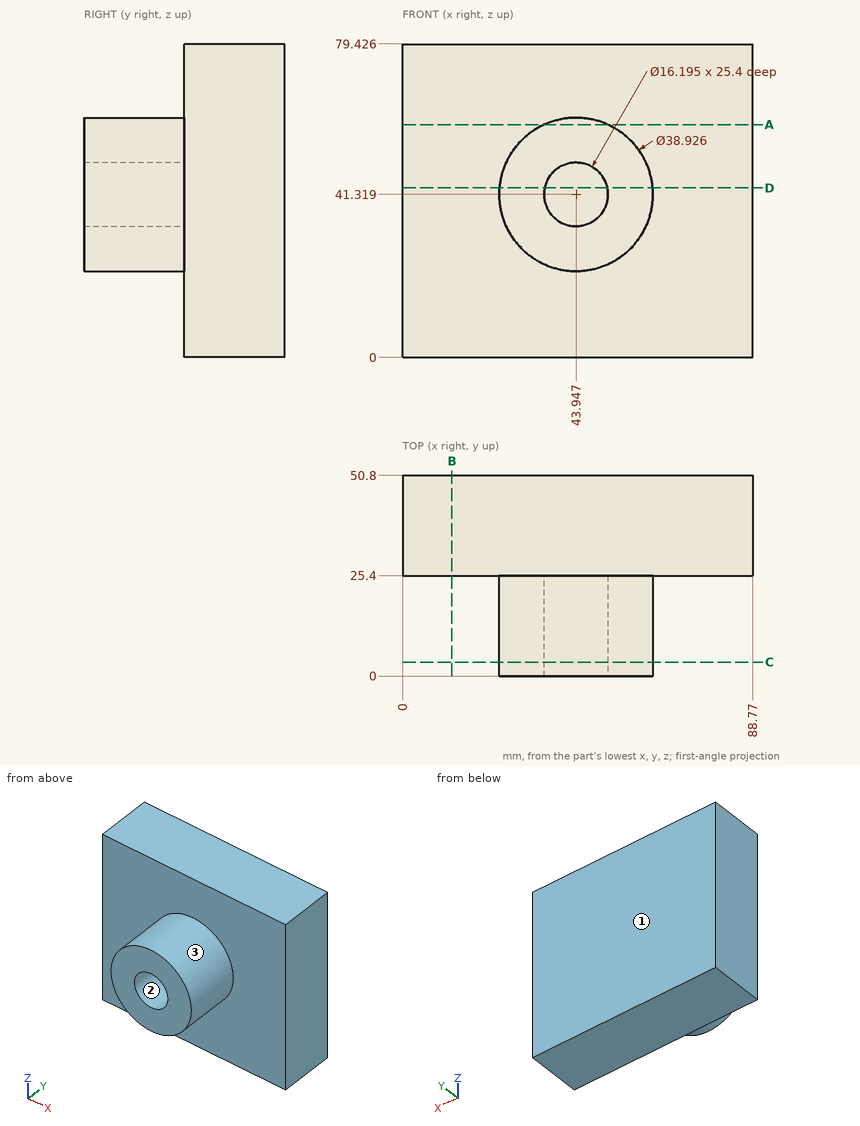
Job drawing, mm, ordinate dimensions from the low corner. One solid piece. Give positions to 0.01 mm unless a question says otherwise; leave off trailing zeros. Loops run counter-clockwise (first coordinate to the right, second up) from the corner with the lowest first, then second, coordinate; pieces in that order, holes last.
Item 1: Pull direction Z, two halves, no side cores. Call the marked faces 1, 2 and 3: released by +Z, released by -Z, zero draft, split by the parting line, or undercut.
Answers follow:
face 1: zero draft
face 2: undercut
face 3: split by the parting line
Item 2: Slice it at D-D, the plane z = 43. List the corners of the cut face in (x, y).
Answers follow:
outline: (0, 25.4) - (24.56, 25.4) - (24.56, 0) - (36.03, 0) - (36.03, 25.4) - (51.87, 25.4) - (51.87, 0) - (63.34, 0) - (63.34, 25.4) - (88.77, 25.4) - (88.77, 50.8) - (0, 50.8) - close
Item 3: Slice it at C-C, the plane y = 3.5. List the corners of the cut face in (x, z) (1 decimal).
Answers follow:
outline: circle Ø38.9 at (43.9, 41.3); hole circle Ø16.2 at (43.9, 41.3)
Item 4: Slice it at B-B, the plane x = 12.5. List the corners of the cut face in (y, z).
Answers follow:
outline: (25.4, 0) - (50.8, 0) - (50.8, 79.43) - (25.4, 79.43) - close
Item 5: Slice it at A-A, the plane z = 59. List the corners of the cut face in (x, y), and give its area (3 significant figures).
Answers follow:
outline: (0, 25.4) - (35.81, 25.4) - (35.81, 0) - (52.08, 0) - (52.08, 25.4) - (88.77, 25.4) - (88.77, 50.8) - (0, 50.8) - close
area: 2,670 mm2
Item 6: Drill centre lines: line 1 (Z direction, x = 44.5, y = 6); line 2 (Y direction, x = 14.5, z = 60); line 3 (X direction, y = 9.5, z = 46.5) (1 decimal). Where is each one in solid material? Low to high.
Answers follow:
line 1: z = 21.86 to 33.24, 49.4 to 60.77
line 2: y = 25.4 to 50.8
line 3: x = 25.2 to 37.7, 50.2 to 62.7
Item 7: Flat gauge pins, fed straight in: pin 1 (6 mm diameter, centred on x = 27.5, z = 59, fed in from -Y); pin 2 (12 mm diameter, centred on x = 30, y = 8, fed in from -Z); pin 3 (1 mm diameter, centred on y = 8, z = 40, fed in from +X); pin 4 (10 mm diameter, centred on y = 13, z = 15.5, fed in from +X). Where does each tip first touch, or does it go through?
Answers follow:
pin 1: stops at y = 25.4
pin 2: stops at z = 23.55
pin 3: stops at x = 63.39
pin 4: passes through
